```python
from build123d import *

# Parameters (mm, degrees)
F0_W     = 268
F0_H     = 84
F0_H_2   = 1400
F0_H_3   = 16
F0_H_4   = 250
F1_DEPTH = 16
F2_DEPTH = 584
F3_W     = 268
F3_H     = 16
F4_DEPTH = 84


with BuildPart() as f1:
    # F0 (on Front) → F1 (new body)
    with BuildSketch(Plane.XZ):
        Polygon((-16, 0), (0, 0), (0, 2048), (-300, 2048), (-300, 0), (-284, 0), (-284, 84), (-16, 84), align=None)
        Polygon((-16, 100), (-284, 100), (-284, 1500), (-284, 1516), (-284, 1766), (-284, 1782), (-284, 2032), (-16, 2032), (-16, 1782), (-16, 1766), (-16, 1516), (-16, 1500), align=None, mode=Mode.SUBTRACT)
        with Locations((-150, 42)):
            Rectangle(F0_W, F0_H)
        with Locations((-150, 800)):
            Rectangle(F0_W, F0_H_2)
        with Locations((-150, 1508)):
            Rectangle(F0_W, F0_H_3)
        with Locations((-150, 1641)):
            Rectangle(F0_W, F0_H_4)
        with Locations((-150, 1774)):
            Rectangle(F0_W, F0_H_3)
        with Locations((-150, 1907)):
            Rectangle(F0_W, F0_H_4)
    extrude(amount=-F1_DEPTH)

    # F0 (on Front) → F2 (join)
    with BuildSketch(Plane.XZ):
        Polygon((-16, 0), (0, 0), (0, 2048), (-300, 2048), (-300, 0), (-284, 0), (-284, 84), (-16, 84), align=None)
        Polygon((-16, 100), (-284, 100), (-284, 1500), (-284, 1516), (-284, 1766), (-284, 1782), (-284, 2032), (-16, 2032), (-16, 1782), (-16, 1766), (-16, 1516), (-16, 1500), align=None, mode=Mode.SUBTRACT)
        with Locations((-150, 1508)):
            Rectangle(F0_W, F0_H_3)
        with Locations((-150, 1774)):
            Rectangle(F0_W, F0_H_3)
    extrude(amount=F2_DEPTH)

    # F3 (on face) → F4 (join, through all)
    with BuildSketch(Plane(origin=(0, 0, 84), x_dir=(1, 0, 0), z_dir=(0, 0, -1))):
        with Locations((-150, 571)):
            Rectangle(F3_W, F3_H)
    extrude(amount=F4_DEPTH)


solid = f1.part
```
Source: CAD feature listing. Evaluate the final solid. Frame: model axes, mm. A direction names the side the tool comes from. Coordinates: 2 decimals unless noted, no trailing zeros. Loops run counter-clockwise (first coordinate to the right, second up) from the corner with the lowest first, then second, coordinate; pieces in that order, holes last. Notation, with made-up numbers: M -7.75,-26.5 L 43.25,-26.5 A12 ccw 43.25,-21.5 Z; hole C 20,-23.75 d9. An arc over 180 degrees is marked long. Use CSV: the item, a comma, the result in double quotes.
(1) Contact query for flat-ended pins moving along their axis: pin 1 (3 mm diameter, centred on x = -166.5, y = -287.5, fed in from -Z); pin 2 (1 mm diameter, centred on y = -357, z = 1421.5, fed in from +X); pin 3 (2 mm diameter, centred on x = -136.5, z = 1657, fed in from -Y). Output: stop coordinate, or through.
Answers follow:
pin 1,"z = 84"
pin 2,"x = 0"
pin 3,"y = 0"
(2) Cut plane C-C on z = 1412.5. Return loops of the section in (x, y), and give its area (3 significant figures).
Answers follow:
outline,"M -300,-584 L -284,-584 L -284,0 L -16,0 L -16,-584 L 0,-584 L 0,16 L -300,16 Z"
area,"23,500 mm²"
(3) Reachability of faces 1 (the face through (-152, -278, 84)), 2 (the face through (0, -280, 1010)), 3 (the face through (-152, 0, 1643)) from +Z, -Z, +X, -X, +Y, -Y: full face, straight path, thin tool, end or side. Return the list, or none.
Answers follow:
face 1,"-Z"
face 2,"+Z, -Z, +X, +Y, -Y"
face 3,"-Y"
(4) Draft query along Y for faces 4 (the face through (-16, -288, 1643)), 5 (the face through (-152, -563, 43)), 6 (the face through (-16, -278, 43)), 7 (the face through (-152, -579, 43)). Return one class per face: pulls with the +Y half, pulls with the -Y half, needs draft (parallel to the pull), parting line crosses it, or undercut.
Answers follow:
face 4,"needs draft"
face 5,"undercut"
face 6,"undercut"
face 7,"pulls with the -Y half"
(5) Line query: line 1 (Z direction, x = -265, y = -82.5); line 2 (X direction, y = -394.5, z = 571.5); line 3 (Y direction, x = -70, z = 1316). Output: solid intervals per line, ascending. Write a range as [from, to].
Answers follow:
line 1,"[84, 100], [1500, 1516], [1766, 1782], [2032, 2048]"
line 2,"[-300, -284], [-16, 0]"
line 3,"[0, 16]"
(6) Cut plane B-B on x = -250. Return loops of the section in (y, z).
Answers follow:
outline,"M -584,84 L -579,84 L -579,0 L -563,0 L -563,84 L 0,84 L 0,0 L 16,0 L 16,2048 L -584,2048 L -584,2032 L 0,2032 L 0,1782 L -584,1782 L -584,1766 L 0,1766 L 0,1516 L -584,1516 L -584,1500 L 0,1500 L 0,100 L -584,100 Z"
(7) Cut plane A-A on y = -125.5. Return loops of the section in (x, z).
Answers follow:
outline,"M -300,0 L -284,0 L -284,84 L -16,84 L -16,0 L 0,0 L 0,2048 L -300,2048 Z; hole M -284,100 L -16,100 L -16,1500 L -284,1500 Z; hole M -284,1516 L -16,1516 L -16,1766 L -284,1766 Z; hole M -284,1782 L -16,1782 L -16,2032 L -284,2032 Z"
